Study the drawing (mm; zero at the part's minimum x, y, z) and answer. A direction names the side the tool comes from. Coordinates: 2 decimals unless noted, no trailing zeros. Write each loop counter-clockwise with the first axis right and the second up, starting at its lowest first coordinate (ties: lowest second). Pieces come first, ordered by that corner, then holes. Notation, with made-up numbers: M 35.25,80.5 L 54.25,80.5 A23 cw 54.25,108.5 Z; hole C 0.25,-4.75 d2. An arc over 180 degrees is marked long. Answer as CSV lines item,"result". Start each with the question number.
(1) For the marked faces 4 and 5, determine the directions among +Z, -Z, +X, -X, +Y, -Y from which every point of the face is accessible in a straight line to the end or side of a thin tool.
(2) A cutting plane is placed at C-C on z = 31. Give the vertices of the cut face in (x, y).
(3) A cutting plane is placed at D-D on y = 25.5. Give the vertices of the cut face in (x, z), then the cut area to 3 significant figures.
(4) The mould has two halves that part along Y. Classify the marked faces 1, 2 and 3: released by +Y, released by -Y, zero draft, split by the parting line, or undercut.
(5) A cutting plane is placed at B-B on x = 109.5. Give the vertices of the cut face in (y, z), then the cut area to 3 significant figures.
(6) A flat-ended cylindrical pin translates along its axis: P1, Ø11.5, axis at y = 75, z = 31, coming from the +X side. Find the tip coordinate at first contact, or state that the pin passes through.
(7) Find the intervals of material crossed by L1, parallel to Z at x = 2, y = 75; L2, parallel to X at y = 139.5, z = 15.5, in increasing order. Write a range as [from, to].
(8) A cutting plane is placed at A-A on y = 75. Give the vertices of the cut face in (x, z).
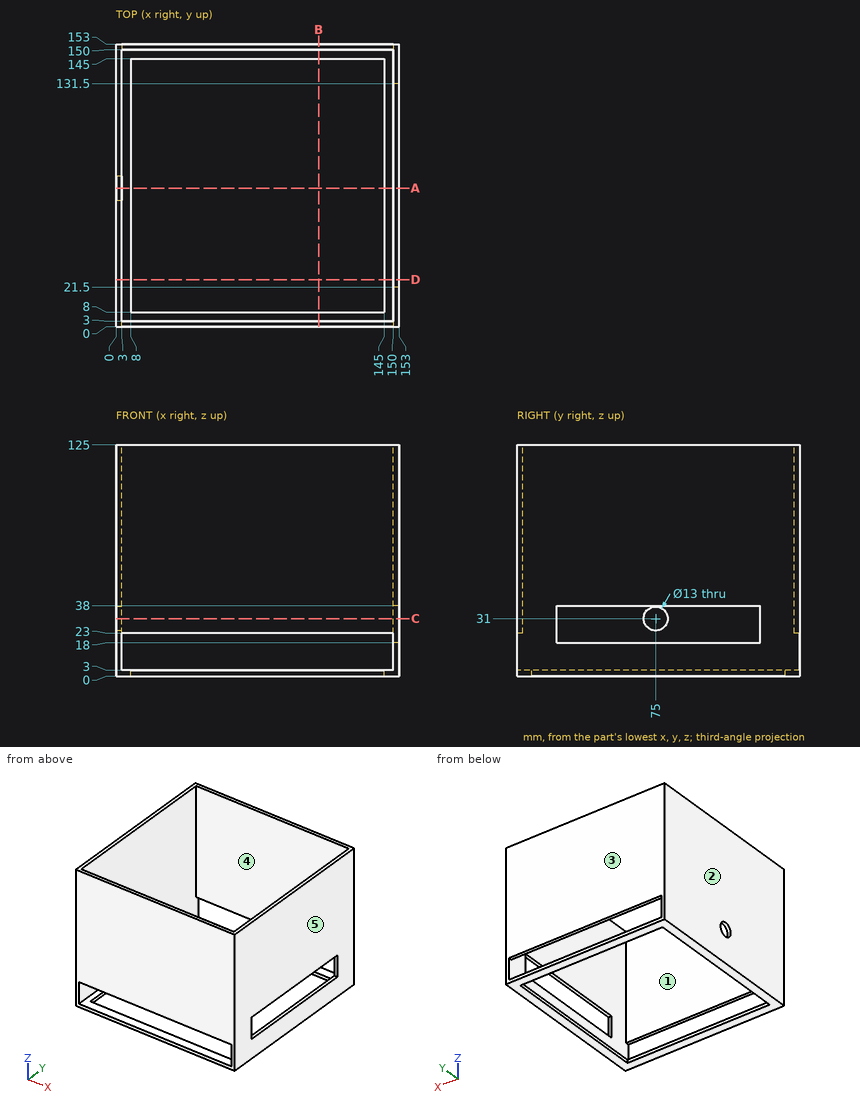
Here are the results:
1,face 4,"+Z"
1,face 5,"+Z, -Z, +X, +Y, -Y"
2,outline,"M 0,0 L 153,0 L 153,21.5 L 150,21.5 L 150,3 L 3,3 L 3,68.5 L 0,68.5 Z; M 0,81.5 L 3,81.5 L 3,150 L 150,150 L 150,131.5 L 153,131.5 L 153,153 L 0,153 Z"
3,outline,"M 0,0 L 8,0 L 8,3 L 3,3 L 3,125 L 0,125 Z; M 145,0 L 153,0 L 153,18 L 150,18 L 150,3 L 145,3 Z; M 150,38 L 153,38 L 153,125 L 150,125 Z"
3,area,"720 mm^2"
4,face 1,"undercut"
4,face 2,"zero draft"
4,face 3,"released by +Y"
5,outline,"M 0,0 L 8,0 L 8,3 L 0,3 Z; M 0,23 L 3,23 L 3,125 L 0,125 Z; M 145,0 L 153,0 L 153,3 L 145,3 Z; M 150,23 L 153,23 L 153,125 L 150,125 Z"
5,area,"660 mm^2"
6,P1,"passes through"
7,L1,"z = [0, 24.5], [37.5, 125]"
7,L2,"x = [0, 3], [150, 153]"
8,outline,"M 0,0 L 8,0 L 8,3 L 3,3 L 3,24.5 L 0,24.5 Z; M 0,37.5 L 3,37.5 L 3,125 L 0,125 Z; M 145,0 L 153,0 L 153,18 L 150,18 L 150,3 L 145,3 Z; M 150,38 L 153,38 L 153,125 L 150,125 Z"
